Could you check a few things on this model? Use its own coordinates, in mm. Give positions to 0.01 mm unless a question says otherwise; leave off trailing zeros. Loops run counter-clockwise (first coordinate to the right, second up) from the corner with the lowest first, then second, coordinate; pieces in that order, holes last. Notation, with made-up numbers: M 88,51 L 106,51 A17 ccw 106,62 Z; hole C 33,5.25 d10. An arc over 180 degrees is marked long. Return JSON: item names as keys, results as strings. Group by question number.
1. If we section it at C-C (z = -24): Write out the boundary of the cut face in (x, y).
2. If we section it at A-A (y = 1): Write out the boundary of the cut face in (x, z), plus the area to 3 significant figures.
3. If we section it at B-B (x = -184): Write out the boundary of the cut face in (y, z), plus the area to 3 significant figures.
4. Please list where these lines run through material, in increasing order: line 1 (X direction, y = 1.75, z = -3); line 2 (Z direction, x = -206.5, y = -3.5); line 3 (Z direction, x = -154, y = -3.5).
5. For pin 1 (2 mm diameter, centred on x = -141, y = 2.5, fed in from -Z); pin 2 (1 mm diameter, centred on x = -132.5, y = 3, fed in from -Z); pin 3 (3 mm diameter, centred on x = -145.5, y = 1, fed in from -Z), each with a flat end and sliding along its axis, tell me the tip position at first contact or that it passes through.
6. If we mould it in two halves opening along Z, with no side actions, what happens to faces 1 (the cylindrical face through (-262.238, 0.053, -85.924)), 2 (the flat face through (-211, -3.81, 2)), 3 (the flat face through (-186.23, -0.05, -64.39))? For each: +Z half, -Z half, draft (parallel to the pull), parting line (faces both ways), or undercut.
```python
from build123d import *

# Parameters (mm, degrees)
F0_R     = 7.62
F1_DEPTH = 3.81
F2_DEPTH = 3.81


with BuildPart() as f1:
    # F0 (on Front) → F1 (new body, symmetric)
    with BuildSketch(Plane.XZ):
        Polygon((-74.70641, 0), (-294.676863, 127), (-294.676863, -127), align=None)
        with Locations((-269.276863, -83.005909)):
            Circle(F0_R, mode=Mode.SUBTRACT)
        with Locations((-269.276863, 83.005909)):
            Circle(F0_R, mode=Mode.SUBTRACT)
        with Locations((-125.50641, 0)):
            Circle(F0_R, mode=Mode.SUBTRACT)
    extrude(amount=F1_DEPTH, both=True)


with BuildPart() as f2:
    # F0 (on Front) → F2 (new body, symmetric)
    with BuildSketch(Plane.XZ):
        with Locations((-269.276863, 83.005909)):
            Circle(F0_R)
        with Locations((-125.50641, 0)):
            Circle(F0_R)
        with Locations((-269.276863, -83.005909)):
            Circle(F0_R)
    extrude(amount=F2_DEPTH, both=True)


with BuildPart() as f1_1:
    add(f1.part)

    # F3: cut F2
    add(f2.part, mode=Mode.SUBTRACT)


solid = f1_1.part
```
Answer:
{
 "1": {"outline": "M -294.68,-3.81 L -116.28,-3.81 L -116.28,3.81 L -294.68,3.81 Z"},
 "2": {"outline": "M -294.68,-127 L -74.71,0 L -294.68,127 Z; hole C -269.28,-83.01 d15.24; hole C -269.28,83.01 d15.24; hole C -125.51,0 d15.24", "area": "27,400 mm²"},
 "3": {"outline": "M -3.81,-63.1 L 3.81,-63.1 L 3.81,63.1 L -3.81,63.1 Z", "area": "962 mm²"},
 "4": {"line 1": "x = -294.68 to -132.51, -118.5 to -79.9", "line 2": "z = -76.09 to 76.09", "line 3": "z = -45.78 to 45.78"},
 "5": {"pin 1": "stops at z = -38.85", "pin 2": "stops at z = -33.66", "pin 3": "stops at z = -41.74"},
 "6": {"face 1": "undercut", "face 2": "draft", "face 3": "-Z half"}
}
